Could you check a few things on this model? Use its own coordinates, in mm. Face numbers are marked on the shaded views. A direction names the side the tool comes from. Coordinates: 2 decimals unless noted, no trailing zeros. Loops run counter-clockwise (first coordinate to the right, second up) from the corner with the lowest first, then second, coordinate; pieces in that order, holes last. Notation, with made-up numbers: (37, 16.5) - (81, 16.5) arc R26 cw to (81, 32.5) - close; hole circle Ø5 at (64.5, -2). An arc over 180 degrees is marked (long way). One line per item, written item: value. Start each with the question number.
(1) If we mould it in two halves opening along X, with no side actions, what happens to the marked faces 4 and 5? For each: pulls with the +X half, pulls with the -X half, needs draft (parallel to the pull), parting line crosses it, or undercut.
(2) On a 3-axis mill with a long thin cutter (end or side, diameter ignored), from which of +Z, -Z, +X, -X, +Y, -Y can I reach the whole of each face in a straight line? I mean the marked faces 1, 2 and 3. Say none if no direction works.
(3) I'm going to push flat-ended pins straight in: P1, Ø5, axis at y = 15, z = -17.5, coming from the +X side; P2, Ø5.5, axis at x = 5, z = -2.5, coming from the +Y side; P3, Ø1, axis at x = 4, z = -83, coming from the +Y side. Where does each tip first touch, or does it pass through?
(4) If we section it at A-A on y = 0: Write out the boundary of the cut face in (x, z), then the cut area to 3 significant figures.
(5) If we section it at B-B on z = -33: Write out the boundary of the cut face in (x, y).
(6) If I drill on line 1 along Y through (x, z) = (0, -12); line 2 along Y through (x, z) = (0, -62.5), over which ranges is the centre line in solid material (lowest first)? Write a range as from..to.
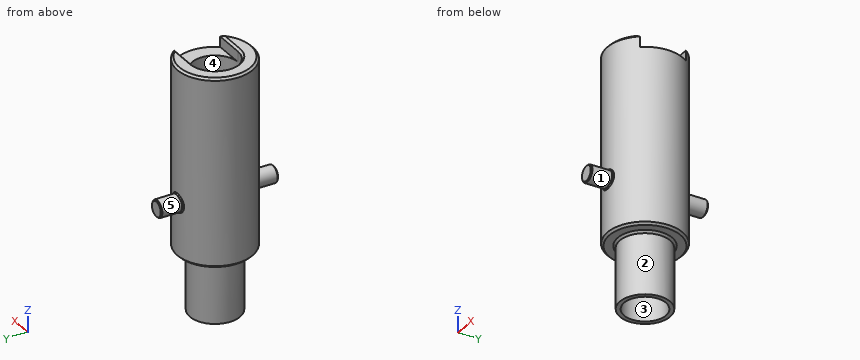
Autodesk Inventor part; units mm, degrees
ref_plane "Plan de construction1" through (0, -18, -45) normal (0, 1, 0) x (-1, 0, 0)
ref_plane "YZ Plane" through (0, 0, 0) normal (1, 0, 0) x (0, 1, 0)
ref_plane "XY Plane" through (0, 0, 0) normal (0, 0, 1) x (1, 0, 0)
sketch "Esquisse3" plane through (0, 0, 0) normal (1, 0, 0) x (0, 1, 0)
  line L0 (17, 0) -> (18, -1)
  line L1 (18, -1) -> (18, -89)
  line L2 (18, -89) -> (17, -90)
  line L3 (17, -90) -> (13, -90)
  line L4 (13, -90) -> (12, -91)
  line L5 (12, -91) -> (12, -120)
  line L6 (12, -120) -> (10, -120)
  line L7 (10, -120) -> (10, -50.25)
  line L8 (11, -50) -> (11, -1)
  line L9 (11, -1) -> (12, 0)
  line L10 (12, 0) -> (17, 0)
  line L11 (0, -144) -> (0, 24)
  line L12 (11, -50) -> (10.25, -50)
  line L13 (10.25, -50) -> (10, -50.25)
  point P0 (0, 0)
  dimension "d4" = 1
  dimension "d5" = 1
  dimension "d6" = 11
  dimension "d7" = 10
  dimension "d8" = 1
  dimension "d9" = 1
  dimension "d10" = 18
  dimension "d11" = 50
  dimension "d12" = 40
  dimension "d13" = 1
  dimension "d14" = 1
  dimension "d16" = 1
  dimension "d17" = 1
  dimension "d18" = 30
  dimension "d20" = 0.25
  dimension "d21" = 0.25
revolve "Révolution1" add sketch "Esquisse3" angle 360 about axis through (0, 0, -10) along (0, 0, 1)
sketch "Esquisse4" plane through (0, 0, 0) normal (1, 0, 0) x (0, 1, 0)
  line L0 (18, -1) -> (18, -89)
  line L1 (18, -89) -> (17, -90)
  line L2 (17, -90) -> (13, -90)
  line L3 (13, -90) -> (12, -91)
  line L4 (12, -91) -> (12, -120)
  line L5 (12, -120) -> (10, -120)
  line L6 (10, -120) -> (10, -50.25)
  line L7 (10, -50.25) -> (10.25, -50)
  line L8 (10.25, -50) -> (11, -50)
  line L9 (11, -50) -> (11, -1)
  line L10 (11, -1) -> (12, 0)
  line L11 (12, 0) -> (17, 0)
  line L12 (17, 0) -> (18, -1)
  line L13 (-18, -89) -> (-18, -1)
  line L14 (-18, -1) -> (-17, 0)
  line L15 (-17, 0) -> (-12, 0)
  line L16 (-12, 0) -> (-11, -1)
  line L17 (-11, -1) -> (-11, -50)
  line L18 (-11, -50) -> (-10.25, -50)
  line L19 (-10.25, -50) -> (-10, -50.25)
  line L20 (-10, -50.25) -> (-10, -120)
  line L21 (-10, -120) -> (-12, -120)
  line L22 (-12, -120) -> (-12, -91)
  line L23 (-12, -91) -> (-13, -90)
  line L24 (-13, -90) -> (-17, -90)
  line L25 (-17, -90) -> (-18, -89)
  line L26 (12, 0) -> (-12, 0)
  line L27 (11, -50) -> (11, -1)
  line L28 (11, -6) -> (-11, -6)
  point P0 (0, 0)
  dimension "d22" = 6
extrude "Extrusion3" cut sketch "Esquisse4" along normal up to surface contours L10 L9 L28 L17 L16 L26
ref_plane "Plan de construction1" through (0, -18, -45) normal (0, 1, 0) x (-1, 0, 0)
sketch "Esquisse5" plane through (0, -18, -45) normal (0, 1, 0) x (-1, 0, 0)
  circle A0 centre (0, -19) radius 4
  line L0 (0, -99) -> (0, 69)
  point P0 (0, 45)
  point P1 (12.0416, 35)
  point P2 (17, 45)
  dimension "d25" = 8
  dimension "d26" = 64
extrude "Extrusion4" add sketch "Esquisse5" along normal blind 2 and the other way blind 10
chamfer "Chanfrein1" distance 0.5 angle 45 4 edges at (-3.0446, -17.7406, -61.4057) (4, -17.5499, -63.9963) (-3.0454, -17.7405, -66.5934) (4, -28, -64)
mirror "Symétrie1" about plane through (0, 0, 0) normal (0, 1, 0) of "Extrusion4", "Chanfrein1"
equation "\"d5\" = d4"
equation "\"d8\" = d4"
equation "\"d9\" = d4"
equation "\"d14\" = d13"
equation "\"d16\" = d13"
equation "\"d17\" = d13"
equation "\"d21\" = d20"
properties part number "canon" material "S235JR (E24-2)"
Values:
1. face 4: undercut
1. face 5: parting line crosses it
2. face 1: -Y
2. face 2: -Z
2. face 3: +Z, -Z
3. P1: stops at x = 12.95
3. P2: stops at y = 17.86
3. P3: stops at y = 17.66
4. outline: (-18, -89) - (-17, -90) - (-13, -90) - (-12, -91) - (-12, -120) - (-10, -120) - (-10, -50.25) - (-10.25, -50) - (-11, -50) - (-11, -1) - (-12, 0) - (-17, 0) - (-18, -1) - close; (10, -120) - (12, -120) - (12, -91) - (13, -90) - (17, -90) - (18, -89) - (18, -6) - (11, -6) - (11, -50) - (10.25, -50) - (10, -50.25) - close
4. area: 1,420 mm2
5. outline: circle Ø36 at (0, 0); hole circle Ø22 at (0, 0)
6. line 1: y = -18..-11, 11..18
6. line 2: y = -28..-10, 10..28
